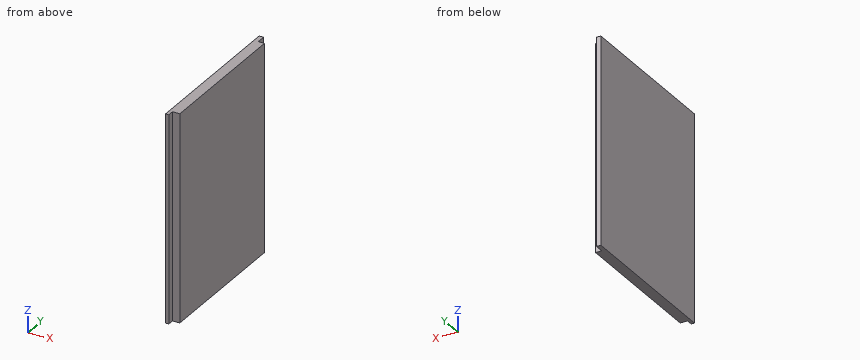
Autodesk Inventor part; units mm, degrees
ref_plane "YZ Plane" through (0, 0, 0) normal (1, 0, 0) x (0, 1, 0)
ref_plane "XZ Plane" through (0, 0, 0) normal (0, 1, 0) x (-1, 0, 0)
ref_plane "XY Plane" through (0, 0, 0) normal (0, 0, 1) x (1, 0, 0)
ref_plane "Work Plane1" through (142.24, 53.9873, -122.2375) normal (0, 0, 1) x (1, 0, 0)
sketch "Sketch1" plane through (142.24, 53.9873, -122.2375) normal (0, 0, 1) x (1, 0, 0)
  line L0 (174.6949, 37.0783) -> (178.6893, 37.0783)
  line L1 (174.6949, -58.3128) -> (174.6949, 37.0783)
  line L2 (178.0128, -58.3128) -> (174.6949, -58.3128)
  line L3 (178.0128, -54.6097) -> (178.0128, -58.3128)
  line L4 (182.3149, -54.6097) -> (178.0128, -54.6097)
  line L5 (182.3149, 31.8435) -> (182.3149, -54.6097)
  line L6 (178.6893, 31.8435) -> (182.3149, 31.8435)
  line L7 (178.6893, 37.0783) -> (178.6893, 31.8435)
  line L8 (181.6164, -53.9112) -> (177.3143, -53.9112)
  line L9 (177.3143, -53.9112) -> (177.3143, -57.6143)
  line L10 (177.3143, -57.6143) -> (175.3934, -57.6143)
  line L11 (175.3934, -57.6143) -> (175.3934, 36.3798)
  line L12 (175.3934, 36.3798) -> (177.9908, 36.3798)
  line L13 (177.9908, 36.3798) -> (177.9908, 31.145)
  line L14 (177.9908, 31.145) -> (181.6164, 31.145)
  line L15 (181.6164, 31.145) -> (181.6164, -53.9112)
  point P0 (-142.24, -53.9873)
  dimension "d0" = 0.6985
extrude "Extrusion1" add sketch "Sketch1" along normal blind 121.92 contours L8 L9 L10 L11 L12 L13 L14 L15
properties part number "Panel"
Could you check a few things on this model? Use its own coordinates, in mm. Round coordinates to 2 decimals unless told otherwise and drop trailing zeros. Write each loop counter-clockwise with the first axis right and the second up, starting at its lowest first coordinate (ties: lowest second). Pieces come first, ordered by that corner, then holes. Notation, with made-up numbers: M -9,29 L 16,29 A6 cw 16,37 Z; hole C -30,84.5 d8. An arc over 180 degrees is marked long. Answer in a Markdown table with one row per item. Add a question column.
Q1. If I drill on line 1 (Y direction, x = 321, z = -28); line 2 (Y direction, x = 319.75, z = -73.5), over which ranges is the centre line in solid material (lowest first)? Write a range as from..to.
Q2. Imagine slicing it at B-B (x = 322.5). Please give me the cut outline in (y, z), then the cut area to 3 significant figures.
Q3. Imagine slicing it at A-A (z = -59). Please give me the cut outline in (x, y), then the cut area to 3 significant figures.
Q4. Will these pins go through, and if not, where does the flat tip stop? pin 1 Ø2.5 at (y, z) = (87.5, -66) entering from +X; pin 2 Ø3 at (y, z) = (-1.5, -62.5) entering from +X.
Values:
| question | item | result |
|---|---|---|
| 1 | line 1 | 0.08..85.13 |
| 1 | line 2 | 0.08..90.37 |
| 2 | outline | M 0.08,-122.24 L 85.13,-122.24 L 85.13,-0.32 L 0.08,-0.32 Z |
| 2 | area | 10,400 mm^2 |
| 3 | outline | M 317.63,-3.63 L 319.55,-3.63 L 319.55,0.08 L 323.86,0.08 L 323.86,85.13 L 320.23,85.13 L 320.23,90.37 L 317.63,90.37 Z |
| 3 | area | 550 mm^2 |
| 4 | pin 1 | x = 320.23 |
| 4 | pin 2 | x = 319.55 |
